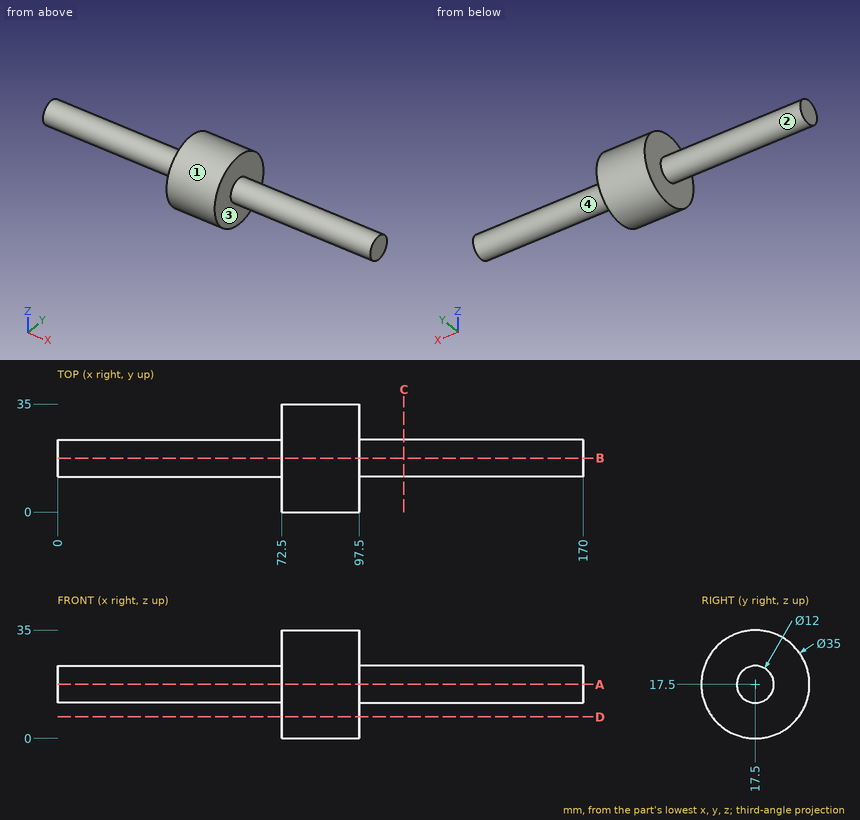
Drawing for the job (mm, zero at the part's lowest x, y, z). A direction names the side the tool comes from. Give positions to 0.01 mm unless a question says otherwise; leave off trailing zeros. Order: outer loops, then holes, each group sorted by start corner. A loop starts at its lowest first (then second) coordinate and runs counter-clockwise, first axis right, second up. Notation, with made-up numbers: (88, 55) - (94, 55) arc R24 cw to (94, 74) - close; hole circle Ø8 at (-39.5, 8.5). An arc over 180 degrees is marked (long way). Write item = value, one per line. Start each with the question number.
1. Cut at D-D, the plane z = 7. List the corners of the cut face in (x, y).
2. Which spindle directions (+Z, -Z, +X, -X, +Y, -Y) get a long thin tool onto all of the face, cutting with end or side? Do the marked faces 1 and 2. Say none if no direction does.
3. Two-plate mould, pull along Y, no slides. Class the marked faces 3 and 4: pulls with the +Y half, pulls with the -Y half, needs draft (parallel to the pull), parting line crosses it, or undercut.
4. Cut at A-A, the plane z = 17.5. List the corners of the cut face in (x, y), and give its area (4 significant figures).
5. Probe line 1 along X through (y, z) = (18.5, 28); line 2 along Y through (x, z) = (52, 17.5); line 3 along Y through (x, z) = (46.5, 16). List the from-to ranges inside material, lowest first.
6. Drop flat-ended pins along their axis: P1, Ø5, axis at x = 52.5, z = 15.5, coming from the +Y side; P2, Ø5, axis at x = 90, y = 5.5, coming from the -Z side; P3, Ø1.5, axis at x = 86.5, y = 11.5, coming from the +Z side. Give the stop position or say it passes through.
7. Cut at C-C, the plane x = 112. List the corners of the cut face in (y, z), and give its area (3 significant figures).
Taken from the geometry:
q1.outline = (72.5, 3.5) - (97.5, 3.5) - (97.5, 31.5) - (72.5, 31.5) - close
q2.face_1 = +X, -X
q2.face_2 = -X
q3.face_3 = needs draft
q3.face_4 = parting line crosses it
q4.outline = (0, 11.5) - (72.5, 11.5) - (72.5, 0) - (97.5, 0) - (97.5, 11.5) - (170, 11.5) - (170, 23.5) - (97.5, 23.5) - (97.5, 35) - (72.5, 35) - (72.5, 23.5) - (0, 23.5) - close
q4.area = 2,615 mm²
q5.line_1 = 72.5 to 97.5
q5.line_2 = 11.5 to 23.5
q5.line_3 = 11.69 to 23.31
q6.P1 = 23.5
q6.P2 = 2.8
q6.P3 = 34.19
q7.outline = circle Ø12 at (17.5, 17.5)
q7.area = 113 mm²
